Could you check a few things on this model? Use its own coordinates, in mm. Give positions to 0.01 mm unless a question says otherwise; leave off trailing zeros. Loops run counter-clockwise (first coordinate to the right, second up) from the corner with the lowest first, then second, coordinate; pieces in that order, holes last.
1. Imagine slicing it at C-C (z = 5.75). Count the separate pieces of the cut face and the enclosed holes in it, plus the area to 3 significant figures.
2. Imagine slicing it at B-B (x = 800). List the corners of the cut face in (y, z) for me.
3. I need wall thicknesses on line 1 along Y through (x, z) = (900, 3); line 2 along X through (y, z) = (-940, 8.25); line 3 along Y through (x, z) = (800, 2.75). Which ranges of each line are inside material? Lowest first, please.
4. For P1, Ø13.5, axis at x = 100, y = -60, coming from the +Z side; P2, Ø5, axis at x = 900, y = -940, coming from the -Z side, each with a flat end and sliding along its axis, tell me the tip position at first contact or that it passes through.
5. Thinking about a two-plate mould opening in Y: for faces 1 (the cylindrical face through (984.964, -14.258, 5.07)), 2 (the flat face through (493, -493, 0)), 3 (the cylindrical face through (14.258, -984.964, 5.07)), 4 (the cylindrical face through (744.722, -449.311, 4.93)), which applies, +Y half, -Y half, draft (parallel to the pull), parting line (faces both ways), or undercut?
6. Imagine slicing it at A-A (y = -500). List the corners of the cut face in (x, z) for me, plus the area to 3 significant figures.
```python
from build123d import *

# Parameters (mm, degrees)
SKETCH_1_W      = 1000
SKETCH_1_H      = 1000
SKETCH_1_R      = 75
SKETCH_1_R_2    = 4.25
EXTRUDE_1_DEPTH = 10
FILLET_1_R      = 50


with BuildPart() as part:
    # 草图1 → 凸台-拉伸1 (new body)
    with BuildSketch(Plane.XY):
        with Locations((500, -500)):
            Rectangle(SKETCH_1_W, SKETCH_1_H)
        with Locations((800, -500)):
            Circle(SKETCH_1_R, mode=Mode.SUBTRACT)
        with Locations((900, -20)):
            Circle(SKETCH_1_R_2, mode=Mode.SUBTRACT)
        with Locations((900, -60)):
            Circle(SKETCH_1_R_2, mode=Mode.SUBTRACT)
        with Locations((860, -20)):
            Circle(SKETCH_1_R_2, mode=Mode.SUBTRACT)
        with Locations((860, -60)):
            Circle(SKETCH_1_R_2, mode=Mode.SUBTRACT)
        with Locations(Location((140, -20, 0), (0, 0, 180))):
            Circle(SKETCH_1_R_2, mode=Mode.SUBTRACT)
        with Locations(Location((100, -20, 0), (0, 0, 180))):
            Circle(SKETCH_1_R_2, mode=Mode.SUBTRACT)
        with Locations(Location((140, -60, 0), (0, 0, 180))):
            Circle(SKETCH_1_R_2, mode=Mode.SUBTRACT)
        with Locations(Location((100, -60, 0), (0, 0, 180))):
            Circle(SKETCH_1_R_2, mode=Mode.SUBTRACT)
        with Locations((100, -980)):
            Circle(SKETCH_1_R_2, mode=Mode.SUBTRACT)
        with Locations((140, -980)):
            Circle(SKETCH_1_R_2, mode=Mode.SUBTRACT)
        with Locations((100, -940)):
            Circle(SKETCH_1_R_2, mode=Mode.SUBTRACT)
        with Locations((140, -940)):
            Circle(SKETCH_1_R_2, mode=Mode.SUBTRACT)
        with Locations(Location((860, -980, 0), (0, 0, 180))):
            Circle(SKETCH_1_R_2, mode=Mode.SUBTRACT)
        with Locations(Location((900, -980, 0), (0, 0, 180))):
            Circle(SKETCH_1_R_2, mode=Mode.SUBTRACT)
        with Locations(Location((860, -940, 0), (0, 0, 180))):
            Circle(SKETCH_1_R_2, mode=Mode.SUBTRACT)
        with Locations(Location((900, -940, 0), (0, 0, 180))):
            Circle(SKETCH_1_R_2, mode=Mode.SUBTRACT)
    extrude(amount=EXTRUDE_1_DEPTH)

    # 圆角1
    fillet_1_edges = [part.edges().sort_by_distance(p)[0] for p in [
        (0, 0, 5),
        (1000, 0, 5),
        (1000, -1000, 5),
        (0, -1000, 5),
    ]]
    fillet(fillet_1_edges, radius=FILLET_1_R)


solid = part.part
```
Derived:
1. separate pieces: 1
1. enclosed holes: 17
1. area: 979,000 mm2
2. outline: (-1000, 0) - (-575, 0) - (-575, 10) - (-1000, 10) - close; (-425, 0) - (0, 0) - (0, 10) - (-425, 10) - close
3. line 1: y = -1000 to -984.25, -975.75 to -944.25, -935.75 to -64.25, -55.75 to -24.25, -15.75 to 0
3. line 2: x = 0 to 95.75, 104.25 to 135.75, 144.25 to 855.75, 864.25 to 895.75, 904.25 to 1000
3. line 3: y = -1000 to -575, -425 to 0
4. P1: stops at z = 10
4. P2: passes through
5. face 1: +Y half
5. face 2: draft
5. face 3: -Y half
5. face 4: undercut
6. outline: (0, 0) - (725, 0) - (725, 10) - (0, 10) - close; (875, 0) - (1000, 0) - (1000, 10) - (875, 10) - close
6. area: 8,500 mm2
